Verification items for this drawing (mm, ordinates from the low corner). Round coordinates to 2 decimals unless told otherwise and drop trailing zeros. Loops run counter-clockwise (first coordinate to the right, second up) from the corner with the lowest first, then second, coordinate; pieces in that order, holes last. Notation, with made-up numbers: (59, 74.25) - (83, 74.25) arc R21 cw to (83, 89.25) - close; hole circle Ø2 at (-27.75, -16). An arc over 180 degrees is marked (long way). Use a Markdown table: item, result. Add a question column.
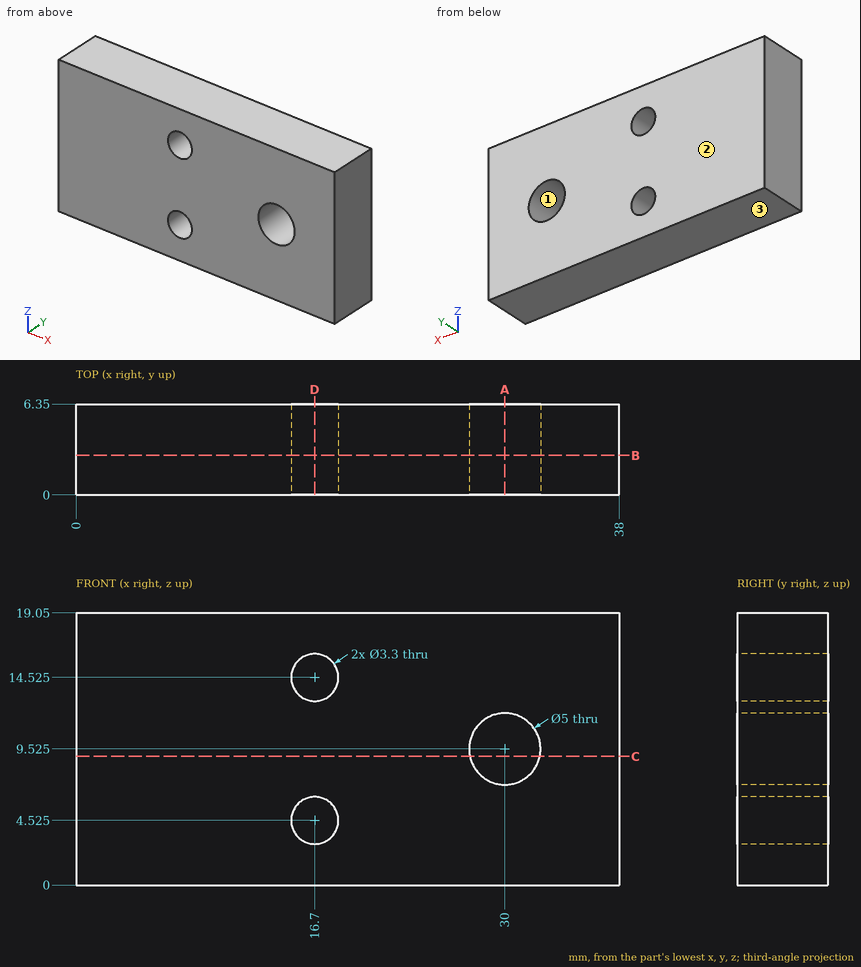
Q1. Section check A-A on x = 30. Record the cut outline in (y, z) (3 decimals).
Q2. Section check C-C on z = 9. Record the cut outline in (x, y).
Q3. Release check for a two-part mould opening along Z. For the marked faces 1, 2 and 3 record: +Z half, -Z half, draft (parallel to the pull), parting line (faces both ways), or undercut.
Q4. Section check D-D on x = 16.7. Record the cut outline in (y, z) (3 decimals).
Q5. Section check B-B on y = 2.75. Record the cut outline in (x, z) (3 decimals), plus the area to 3 significant figures.
Q6. Thickness scan on line 1 along X through (y, z) = (2.25, 4.5); line 2 along Z through (x, y) = (16, 5); line 3 along Z through (x, y) = (16.5, 6.25). Record the ranges inside material, lowest first.
Q7. Go/stop test with a flat-tipped pin: pin 1 Ø2 at (x, z) = (16.7, 4.525) entering from -Y. Record where the tip stops, or that it passes through.
Determined:
| question | item | result |
|---|---|---|
| 1 | outline | (0, 0) - (6.35, 0) - (6.35, 7.025) - (0, 7.025) - close; (0, 12.025) - (6.35, 12.025) - (6.35, 19.05) - (0, 19.05) - close |
| 2 | outline | (0, 0) - (27.56, 0) - (27.56, 6.35) - (0, 6.35) - close; (32.44, 0) - (38, 0) - (38, 6.35) - (32.44, 6.35) - close |
| 3 | face 1 | undercut |
| 3 | face 2 | draft |
| 3 | face 3 | -Z half |
| 4 | outline | (0, 0) - (6.35, 0) - (6.35, 2.875) - (0, 2.875) - close; (0, 6.175) - (6.35, 6.175) - (6.35, 12.875) - (0, 12.875) - close; (0, 16.175) - (6.35, 16.175) - (6.35, 19.05) - (0, 19.05) - close |
| 5 | outline | (0, 0) - (38, 0) - (38, 19.05) - (0, 19.05) - close; hole circle Ø3.3 at (16.7, 4.525); hole circle Ø3.3 at (16.7, 14.525); hole circle Ø5 at (30, 9.525) |
| 5 | area | 687 mm² |
| 6 | line 1 | x = 0 to 15.05, 18.35 to 38 |
| 6 | line 2 | z = 0 to 3.03, 6.02 to 13.03, 16.02 to 19.05 |
| 6 | line 3 | z = 0 to 2.89, 6.16 to 12.89, 16.16 to 19.05 |
| 7 | pin 1 | passes through |
